Could you check a few things on this model? Use its own coordinates, in mm. A direction names the side the tool comes from. Coordinates: 2 decimals unless noted, no trailing zeros. Loops run counter-clockwise (first coordinate to the right, second up) from the corner with the lowest first, then second, coordinate; pieces in that order, holes last. Notation, with made-up numbers: M 11.25,74 L 15.25,74 A13 cw 15.25,79 Z; hole C -37.75,16 d7. An arc over 180 degrees is marked long. Write each question's results on one line, items separated by ' | '.
```python
from build123d import *

# Parameters (mm, degrees)
SKETCH1_W                   = 50.8
SKETCH1_H                   = 203.2
BOSS_EXTRUDE1_DEPTH         = 12.7
F_1_4_20_TAPPED_HOLE1_D     = 5.1054
F_1_4_20_TAPPED_HOLE1_DEPTH = 25.4
F_1_4_20_TAPPED_HOLE1_TIP   = 1.533816902
SKETCH4_R                   = 6.35
CUT_EXTRUDE1_DEPTH          = 13.7


with BuildPart() as part:
    # Sketch1 → Boss-Extrude1 (new body)
    with BuildSketch(Plane.XY):
        with Locations((0, 101.6)):
            Rectangle(SKETCH1_W, SKETCH1_H)
    extrude(amount=BOSS_EXTRUDE1_DEPTH)

    # 1/4-20 Tapped Hole1
    with Locations(Plane(origin=(0, 0, 0), x_dir=(-1, 0, 0), z_dir=(0, -1, 0))):
        with Locations((15.875, -6.35), (-15.875, -6.35)):
            Hole(F_1_4_20_TAPPED_HOLE1_D / 2, depth=F_1_4_20_TAPPED_HOLE1_DEPTH)
            with Locations((0, 0, -(F_1_4_20_TAPPED_HOLE1_DEPTH + F_1_4_20_TAPPED_HOLE1_TIP / 2))):  # 118° drill point
                Cone(0, F_1_4_20_TAPPED_HOLE1_D / 2, F_1_4_20_TAPPED_HOLE1_TIP, mode=Mode.SUBTRACT)

    # Sketch4 → Cut-Extrude1 (cut, through all)
    with BuildSketch(Plane(origin=(0, 0, 0), x_dir=(-1, 0, 0), z_dir=(0, 0, -1))):
        with Locations((0, 184.15)):
            Circle(SKETCH4_R)
    extrude(amount=-CUT_EXTRUDE1_DEPTH, mode=Mode.SUBTRACT)


solid = part.part
```
(1) Will these pins go through, and if not, where does the flat tip stop? P1, Ø3, axis at x = -15.875, z = 6.35, coming from the -Y side; P2, Ø7.5, axis at x = 0, y = 184.15, coming from the -Z side.
Reported:
P1: stops at y = 26.03 | P2: passes through
(2) Imagine slicing it at C-C, the plane y = 18. List the corners of the cut face in (x, z) for me (3 decimals).
Reported:
outline: M -25.4,0 L 25.4,0 L 25.4,12.7 L -25.4,12.7 Z; hole C -15.875,6.35 d5.105; hole C 15.875,6.35 d5.105
(3) Imagine slicing it at B-B, the plane y = 184.15. List the corners of the cut face in (x, z) for me, and give its area (3 significant figures).
Reported:
outline: M -25.4,0 L -6.35,0 L -6.35,12.7 L -25.4,12.7 Z; M 6.35,0 L 25.4,0 L 25.4,12.7 L 6.35,12.7 Z | area: 484 mm2
(4) If we mould it in two halves opening along Z, with no side actions, what happens to faces 3 (the flat face through (0, 103, 12.7)), 4 (the cylindrical face through (1.38, 177.95, 6.26)), 5 (the conical face through (16.318, 26.667, 6.331))? For each: released by +Z, released by -Z, zero draft, split by the parting line, or undercut.
Reported:
face 3: released by +Z | face 4: zero draft | face 5: undercut
(5) Please list where these lines run through material, in increasing order: probe 1 along Y at (x, z) = (0, 9.5); probe 2 along X at (y, z) = (183.5, 1.25); probe 3 along Y at (x, z) = (4, 5.25). Write a range as from..to.
Reported:
probe 1: y = 0..177.8, 190.5..203.2 | probe 2: x = -25.4..-6.32, 6.32..25.4 | probe 3: y = 0..179.22, 189.08..203.2
(6) Which directions (+Z, -Z, +X, -X, +Y, -Y) give clear straight access to the entire face, cutting with the end or side of a thin tool? Please do faces 1 (the cylindrical face through (-13.44, 12.88, 5.58)), 2 (the flat face through (0, 103, 0)).
Reported:
face 1: -Y | face 2: -Z, +X, -X, +Y, -Y
(7) Imagine slicing it at A-A, the plane x = 0. List the corners of the cut face in (y, z) for me.
Reported:
outline: M 0,0 L 177.8,0 L 177.8,12.7 L 0,12.7 Z; M 190.5,0 L 203.2,0 L 203.2,12.7 L 190.5,12.7 Z
